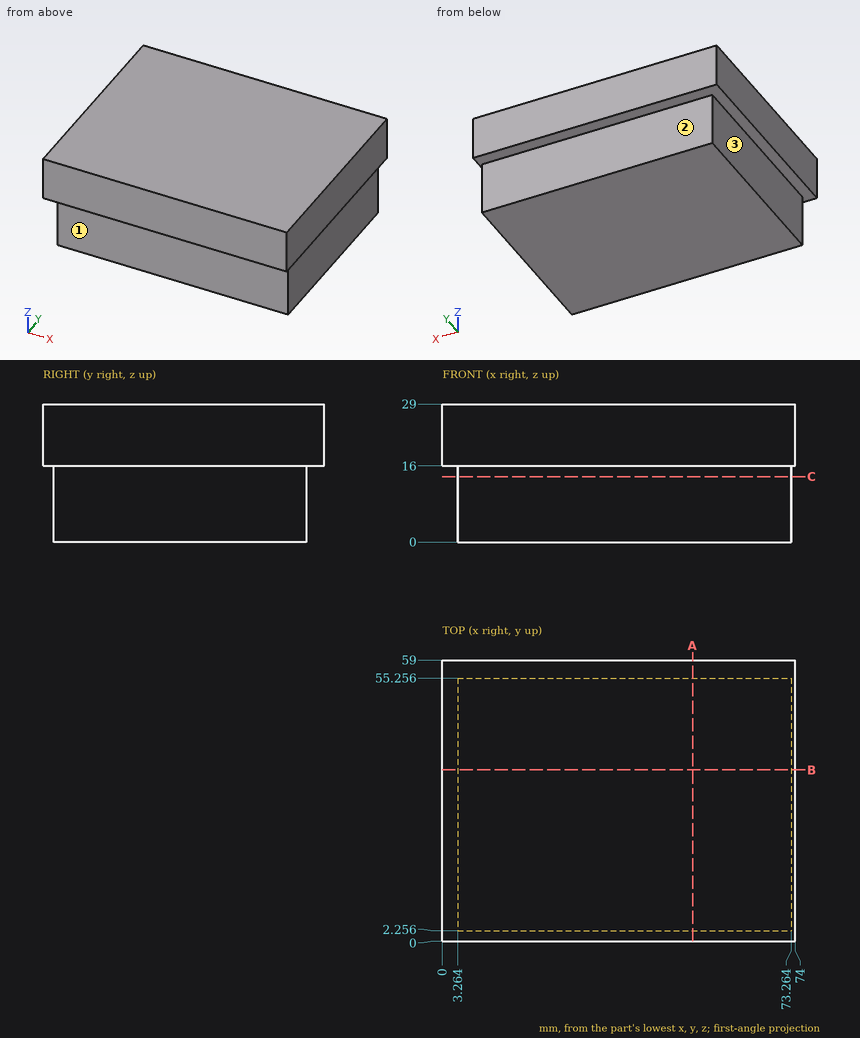
Source: three-view drawing plus pictorial views. Frame: mm from the lowest corner of the part. A direction names the side the tool comes from. Round coordinates to 2 decimals unless told otherwise and drop trailing zeros. Loops run counter-clockwise (first coordinate to the right, second up) from the corner with the lowest first, then second, coordinate; pieces in that order, holes last. Notation, with made-up numbers: M 23.5,42.25 L 75.5,42.25 A12 cw 75.5,52.25 Z; hole C 18,77.25 d4. An arc over 180 degrees is marked long. Answer as CSV lines item,"result". Start each with the question number.
(1) Section A-A, the plane x = 52.5. Output: boundary loops of the cut face in (y, z), plus the area to 4 significant figures.
(2) Section B-B, the plane y = 36. Output: boundary loops of the cut face in (x, z).
(3) First-contact query: pin 1 (17.5 mm diameter, centred on x = 48.5, y = 33, fed in from -Z); pin 2 (13 mm diameter, centred on y = 38, z = 9, fed in from +X); pin 3 (8 mm diameter, centred on x = 46.5, z = 8, fed in from -Y); pin 4 (8 mm diameter, centred on x = 29, z = 11.5, fed in from +Y). Flat tips, straight axial feed; report the tip coordinate or a pass-through.
(4) Section C-C, the plane z = 13.75. Output: boundary loops of the cut face in (x, y), plus the area to 3 significant figures.
(5) Line query: line 1 (Y direction, x = 55, z = 4.25); line 2 (X direction, y = 10, z = 4.75). Output: solid intervals per line, ascending. Write a range as [from, to].
(6) Reachability of the marked faces 1, 2 and 3 from +Z, -Z, +X, -X, +Y, -Y: full face, straight path, thin tool, end or side. Return the list, or none.
Values found:
1,outline,"M 0,16 L 2.26,16 L 2.26,0 L 55.26,0 L 55.26,16 L 59,16 L 59,29 L 0,29 Z"
1,area,"1,615 mm²"
2,outline,"M 0,16 L 3.26,16 L 3.26,0 L 73.26,0 L 73.26,16 L 74,16 L 74,29 L 0,29 Z"
3,pin 1,"stops at z = 0"
3,pin 2,"stops at x = 73.26"
3,pin 3,"stops at y = 2.26"
3,pin 4,"stops at y = 55.26"
4,outline,"M 3.26,2.26 L 73.26,2.26 L 73.26,55.26 L 3.26,55.26 Z"
4,area,"3,710 mm²"
5,line 1,"y = [2.26, 55.26]"
5,line 2,"x = [3.26, 73.26]"
6,face 1,"-Z, +X, -X, -Y"
6,face 2,"-Z, +X, -X, +Y"
6,face 3,"-Z, -X, +Y, -Y"
